from build123d import *

# Parameters (mm, degrees)
SKETCH1_R           = 12.7
SKETCH1_R_2         = 6.985
BOSS_EXTRUDE1_DEPTH = 2.54
BOSS_EXTRUDE2_START = -7.62
SKETCH1_3_R         = 9.525
SKETCH1_3_R_2       = 6.985
BOSS_EXTRUDE2_DEPTH = 7.62
FILLET1_R           = 1.27
FILLET2_R           = 0.762


with BuildPart() as part:
    # Sketch1 → Boss-Extrude1 (new body)
    with BuildSketch(Plane(origin=(0, 0, 0), x_dir=(1, 0, 0), z_dir=(0, 1, 0))):
        with Locations(Location((0, 0, 0), (0, 0, 270))):
            Circle(SKETCH1_R)
        with Locations(Location((0, 0, 0), (0, 0, 270))):
            Circle(SKETCH1_R_2, mode=Mode.SUBTRACT)
    extrude(amount=BOSS_EXTRUDE1_DEPTH)

    # Sketch1_3 → Boss-Extrude2 (add)
    with BuildSketch(Plane(origin=(0, 0, 0), x_dir=(1, 0, 0), z_dir=(0, 1, 0)).offset(BOSS_EXTRUDE2_START)):
        with Locations(Location((0, 0, 0), (0, 0, 270))):
            Circle(SKETCH1_3_R)
        with Locations(Location((0, 0, 0), (0, 0, 270))):
            Circle(SKETCH1_3_R_2, mode=Mode.SUBTRACT)
    extrude(amount=BOSS_EXTRUDE2_DEPTH)

    # Fillet1
    fillet1_edges = [part.edges().sort_by_distance(p)[0] for p in [
        (0, 2.54, -6.985),
    ]]
    fillet(fillet1_edges, radius=FILLET1_R)

    # Fillet2
    fillet2_edges = [part.edges().sort_by_distance(p)[0] for p in [
        (0, 0, -9.525),
    ]]
    fillet(fillet2_edges, radius=FILLET2_R)

    # Sketch2 → Revolve1 (revolve)
    with BuildSketch(Plane(origin=(0, 0, 0), x_dir=(0, 0, -1), z_dir=(1, 0, 0)), mode=Mode.PRIVATE) as revolve1_sk:
        with BuildLine():
            Line((9.525, -6.35), (9.525, -7.62))
            ThreePointArc((9.525, -7.62), (9.695147737, -6.985), (9.525, -6.35))
        make_face()
    revolve(revolve1_sk.sketch.rotate(Axis((0, 3.048, 0), (0, -1, 0)), 180), axis=Axis((0, 3.048, 0), (0, -1, 0)))


solid = part.part
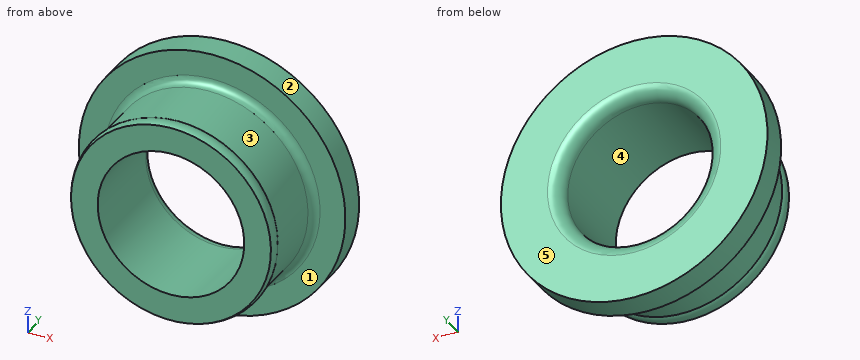
Verification items for the finished model (mm, model axes). Face numbers are marked on the shaded views. A direction names the side the tool comes from. Give positions to 0.01 mm unless a question says otherwise; leave off trailing zeros. Loops run counter-clockwise (first coordinate to the right, second up) from the corner with the lowest first, then second, coordinate; pieces in that order, holes last. Notation, with made-up numbers: (71, 36.5) - (83, 36.5) arc R23 ccw to (83, 73.5) - close; hole circle Ø6 at (2, -33). An arc over 180 degrees is marked (long way). Write item = value, one per line. Start each with the question number.
Q1. Tool access check on the marked faces 1 and 2. Record the directions out of +Z, -Z, +X, -X, +Y, -Y that give a thin tool (end or side, any length) a straight path to the whole face; none if there is none.
Q2. Cross-section at D-D, the plane x = 10.75. Enter the section's corners in (y, z).
Q3. Mould release check, pull along Z, two halves, no side actions. Record for the marked faces 3, 4 and 5: released by +Z, released by -Z, zero draft, split by the parting line, or undercut.
Q4. Cross-section at C-C, the plane y = -4.5. Enter the section's corners in (x, z) (3 decimals).
Q5. Depth check by flat-ended pin: P1, Ø3, axis at y = -2.5, z = 5, coming from the -X side; P2, Ø4, axis at x = -5.5, y = -5.5, coming from the +Z side; P3, Ø6, axis at x = -8, y = -4, coming from the +Z side; P4, Ø1.5, axis at x = 5, z = -3, coming from the -Y side. Enter the tip coordinate at first touch or a pass-through.
Q6. Thickness scan on line 1 (X direction, y = -1.75, z = 0) (3 decimals); line 2 (X direction, y = -2, z = 5.5); line 3 (Y direction, x = 7.5, z = -6). Record the ranges inside material, lowest first.
Q7. Cross-section at A-A, the plane z = 0. Enter the section's corners in (x, y) (3 decimals), and give its area (3 significant figures).
Q8. Cross-section at B-B, the plane x = 0. Enter the section's corners in (y, z) (3 decimals), and give its area (3 significant figures).
Answer key:
q1.face_1 = -Y
q1.face_2 = +Y, -Y
q2.outline = (0, -6.76) - (2.54, -6.76) - (2.54, 6.76) - (0, 6.76) - close
q3.face_3 = split by the parting line
q3.face_4 = undercut
q3.face_5 = zero draft
q4.outline = circle Ø19.05 at (0, 0); hole circle Ø13.97 at (0, 0)
q5.P1 = -8.86
q5.P2 = 8.86
q5.P3 = 8.11
q5.P4 = through
q6.line_1 = -9.525 to -6.985, 6.985 to 9.525
q6.line_2 = -7.78 to -4.31, 4.31 to 7.78
q6.line_3 = -7.46 to -6.51, -0.42 to 2.54
q7.outline = (-12.7, 0) - (-10.287, 0) arc R0.762 cw to (-9.525, -0.762) - (-9.525, -6.35) arc R1.27 ccw to (-9.525, -7.62) - (-6.985, -7.62) - (-6.985, 1.27) arc R1.27 ccw to (-8.255, 2.54) - (-12.7, 2.54) - close; (6.985, -7.62) - (9.525, -7.62) arc R1.27 ccw to (9.525, -6.35) - (9.525, -0.762) arc R0.762 cw to (10.287, 0) - (12.7, 0) - (12.7, 2.54) - (8.255, 2.54) arc R1.27 ccw to (6.985, 1.27) - close
q7.area = 67.6 mm^2
q8.outline = (-7.62, -9.525) arc R1.27 ccw to (-6.35, -9.525) - (-0.762, -9.525) arc R0.762 cw to (0, -10.287) - (0, -12.7) - (2.54, -12.7) - (2.54, -8.255) arc R1.27 ccw to (1.27, -6.985) - (-7.62, -6.985) - close; (-7.62, 6.985) - (1.27, 6.985) arc R1.27 ccw to (2.54, 8.255) - (2.54, 12.7) - (0, 12.7) - (0, 10.287) arc R0.762 cw to (-0.762, 9.525) - (-6.35, 9.525) arc R1.27 ccw to (-7.62, 9.525) - close
q8.area = 67.6 mm^2
